```python
from build123d import *

# Parameters (mm, degrees)
BOSS_EXTRUDE11_DEPTH = 1.5
BOSS_EXTRUDE12_START = 10
BOSS_EXTRUDE12_DEPTH = 10
BOSS_EXTRUDE15_START = 11.5
BOSS_EXTRUDE15_DEPTH = 1.5


with BuildPart() as part:
    # base → Boss-Extrude11 (new body)
    with BuildSketch(Plane(origin=(0, 0, 0), x_dir=(1, 0, 0), z_dir=(0, 1, 0))):
        with BuildLine():
            Line((-2.5, 14), (-2.5, 22.612220148))
            ThreePointArc((-2.5, 22.612220148), (0, -22.75), (2.5, 22.612220148))
            Line((2.5, 22.612220148), (2.5, 14))
            ThreePointArc((2.5, 14), (0, 11.5), (-2.5, 14))
        make_face()
    extrude(amount=-BOSS_EXTRUDE11_DEPTH)

    # rim → Boss-Extrude12 (add)
    with BuildSketch(Plane(origin=(0, 0, 0), x_dir=(1, 0, 0), z_dir=(0, 1, 0)).offset(BOSS_EXTRUDE12_START)):
        with BuildLine():
            Line((2.5, 22.612220148), (2.5, 14))
            ThreePointArc((2.5, 14), (0, 11.5), (-2.5, 14))
            Line((-2.5, 14), (-2.5, 22.612220148))
            ThreePointArc((-2.5, 22.612220148), (0, -22.75), (2.5, 22.612220148))
        make_face()
        with BuildLine():
            Line((-3.5, 21.446457505), (-3.5, 14))
            ThreePointArc((-3.5, 14), (0, 10.5), (3.5, 14))
            Line((3.5, 14), (3.5, 21.446457505))
            ThreePointArc((3.5, 21.446457505), (0, -21.730175782), (-3.5, 21.446457505))
        make_face(mode=Mode.SUBTRACT)
    extrude(amount=-BOSS_EXTRUDE12_DEPTH)

    # lid → Boss-Extrude15 (add)
    with BuildSketch(Plane(origin=(0, 0, 0), x_dir=(1, 0, 0), z_dir=(0, 1, 0)).offset(BOSS_EXTRUDE15_START)):
        with BuildLine():
            Line((-2.5, 14), (-2.5, 29))
            ThreePointArc((-2.5, 29), (0, -29.107559156), (2.5, 29))
            Line((2.5, 29), (2.5, 14))
            ThreePointArc((2.5, 14), (0, 11.5), (-2.5, 14))
        make_face()
        with BuildLine():
            ThreePointArc((-3.5, 21.446457505), (0, -21.730175782), (3.5, 21.446457505))
            Line((3.5, 21.446457505), (3.5, 14))
            ThreePointArc((3.5, 14), (0, 10.5), (-3.5, 14))
            Line((-3.5, 14), (-3.5, 21.446457505))
        make_face(mode=Mode.SUBTRACT)
    extrude(amount=-BOSS_EXTRUDE15_DEPTH)


solid = part.part
```
The model under review builds one solid part; all positions refer to its coordinate system, in mm. A direction names the side the tool comes from. Round coordinates to 2 decimals unless told otherwise and drop trailing zeros. Loops run counter-clockwise (first coordinate to the right, second up) from the corner with the lowest first, then second, coordinate; pieces in that order, holes last. Notation, with made-up numbers: (82.5, 20) - (103.5, 20) arc R12 cw to (103.5, 32) - close; hole circle Ø9 at (-27, 23.5). An arc over 180 degrees is marked (long way). Use a Markdown table: item, result. Add a question column.
Q1. Add section B-B (x = 0). State the section outline as (y, z) points.
Q2. Add section D-D (x = -10.5). State the section outline as (y, z) points (3 decimals).
Q3. The part is to be moulded in two halves that separate along Z. For faces 4 (the face through (-4.45, 11.5, 21.44)), 5 (the face through (-0.1, 5.8, -10.5)), 6 (the face through (-1.24, 10.76, 29.08)), say which applies: pulls with the +Z half, pulls with the -Z half, needs draft (parallel to the pull), parting line crosses it, or undercut.
Q4. Insertion check: pin 1 Ø6 at (y, z) = (7.5, -18.5) entering from +X; pin 2 Ø1 at (x, y) = (-13.5, 5) entering from -Z; pin 3 Ø1 at (x, z) = (1, 20.5) entering from +Y. Each pin has a flat end and moves straight along its axis. Give the tip position at first contact, or say it passes through.
Q5. Machinability: for faces 1 (the face through (-2.5, 5, -18)), 2 (the face through (3.5, 6, -18)), 3 (the face through (0, 10, 24)), which of the approach directions +Z, -Z, +X, -X, +Y, -Y give a long, thin tool a straight path to every point of the face, cutting with its end or side? Answer none if there is none.
Q6. For probe 1 along X at (y, z) = (10.7, 0); probe 2 along X at (y, z) = (3, 0); probe 3 along X at (y, z) = (2.5, -16), list the stretches that pass through material, from the lowest coordinate up.
Q7. Add section C-C (z = 0). State the section outline as (x, y) points.
Q8. Add section A-A (y = 6). State the section outline as (x, z) points, plus the area to 3 significant figures.
Worked answers:
| question | item | result |
|---|---|---|
| 1 | outline | (-1.5, -11.5) - (11.5, -11.5) - (11.5, -10.5) - (0, -10.5) - (0, 21.73) - (11.5, 21.73) - (11.5, 29.11) - (10, 29.11) - (10, 22.75) - (-1.5, 22.75) - close |
| 2 | outline | (-1.5, -20.182) - (10, -20.182) - (10, -27.148) - (11.5, -27.148) - (11.5, -19.025) - (0, -19.025) - (0, 19.025) - (11.5, 19.025) - (11.5, 27.148) - (10, 27.148) - (10, 20.182) - (-1.5, 20.182) - close |
| 3 | face 4 | needs draft |
| 3 | face 5 | undercut |
| 3 | face 6 | parting line crosses it |
| 4 | pin 1 | x = 23.74 |
| 4 | pin 2 | z = -18.67 |
| 4 | pin 3 | y = 0 |
| 5 | face 1 | -Z, +Y, -Y |
| 5 | face 2 | +Y |
| 5 | face 3 | -Y |
| 6 | probe 1 | -29.11 to -21.73, 21.73 to 29.11 |
| 6 | probe 2 | -22.75 to -21.73, 21.73 to 22.75 |
| 6 | probe 3 | -16.17 to -14.7, -3.5 to -2.5, 2.5 to 3.5, 14.7 to 16.17 |
| 7 | outline | (-29.11, 10) - (-22.75, 10) - (-22.75, -1.5) - (22.75, -1.5) - (22.75, 10) - (29.11, 10) - (29.11, 11.5) - (21.73, 11.5) - (21.73, 0) - (-21.73, 0) - (-21.73, 11.5) - (-29.11, 11.5) - close |
| 8 | outline | (-2.5, -22.61) - (-2.5, -14) arc R2.5 cw to (2.5, -14) - (2.5, -22.61) arc R22.75 ccw (long way) to start; hole (-3.5, -21.45) - (-3.5, -14) arc R3.5 cw to (3.5, -14) - (3.5, -21.45) arc R21.73 ccw (long way) to start |
| 8 | area | 162 mm² |
